Could you check a few things on this model? Use its own coordinates, in mm. Round coordinates to 2 decimals unless told otherwise and drop trailing zeros. Loops run counter-clockwise (first coordinate to the right, second up) from the corner with the lowest first, then second, coordinate; pieces in that order, holes last. Notation, with made-up numbers: (-23.5, 85) -> (13.5, 85) arc R34 ccw to (13.5, 116) -> close; hole circle Ø6 at (28, 87). An arc over 180 degrees is marked (long way). One line per item, written item: value.
Autodesk Inventor part; units mm, degrees
ref_plane "YZ Plane" through (0, 0, 0) normal (1, 0, 0) x (0, 1, 0)
ref_plane "XZ Plane" through (0, 0, 0) normal (0, 1, 0) x (-1, 0, 0)
ref_plane "XY Plane" through (0, 0, 0) normal (0, 0, 1) x (1, 0, 0)
sketch "Sketch1" plane through (0, 0, 0) normal (0, 1, 0) x (-1, 0, 0)
  line L0 (0, 0) -> (0, -190) construction
  line L1 (4, 0) -> (4, -190)
  line L2 (-4, -190) -> (-4, 0)
  arc A0 (4, 0) -> (-4, 0) centre (0, 0) ccw
  arc A1 (-4, -190) -> (4, -190) centre (0, -190) ccw
  circle A2 centre (0, 0) radius 2.1
  circle A3 centre (0, -190) radius 2.1
  point P0 (0, -95)
  dimension "d0" = 190
  dimension "d1" = 8
  dimension "d2" = 4.2
  dimension "d3" = 4.2
extrude "Extrusion1" add sketch "Sketch1" along normal blind 5
(1) Thinking about a two-plate mould opening in X: for faces 1 (the face through (0, 0, -94)), 2 (the face through (0.273, 2.465, -192.082)), 3 (the face through (-4, 2, -94)), 4 (the face through (0, 2, 4)), which applies, released by +X, released by -X, zero draft, split by the parting line, or undercut?
Recorded:
face 1: zero draft
face 2: undercut
face 3: released by -X
face 4: split by the parting line
(2) If I drill on L1, parallel to Z at x = 0, y = 2.3; L2, parallel to Z at x = 1.5, y = 3.45; L3, parallel to X at y = 4.05, z = -190, over which ranges is the centre line in solid material (lowest first)?
Recorded:
L1: -194 to -192.1, -187.9 to -2.1, 2.1 to 4
L2: -193.71 to -191.47, -188.53 to -1.47, 1.47 to 3.71
L3: -4 to -2.1, 2.1 to 4
(3) If we section it at A-A, the plane x = 0: Please give me the cut outline in (y, z).
Recorded:
outline: (0, -194) -> (5, -194) -> (5, -192.1) -> (0, -192.1) -> close; (0, -187.9) -> (5, -187.9) -> (5, -2.1) -> (0, -2.1) -> close; (0, 2.1) -> (5, 2.1) -> (5, 4) -> (0, 4) -> close
(4) If we section it at B-B, the plane y = 0.85: Please give me the cut outline in (x, z), then the cut area to 3 significant figures.
Recorded:
outline: (-4, -190) arc R4 ccw to (4, -190) -> (4, 0) arc R4 ccw to (-4, 0) -> close; hole circle Ø4.2 at (0, -190); hole circle Ø4.2 at (0, 0)
area: 1,540 mm²
(5) I'm going to push a flat-ended pin straight in: pin 1 Ø2 at (x, y) = (-3, 4.5) entering from -Z. Where does the tip first touch, or does it pass through?
Recorded:
pin 1: z = -193.46
